Verification items for the finished model (mm, model axes). A direction names the side the tool comes from. Coordinates: 2 decimals unless noted, no trailing zeros. Write each loop counter-clockwise with the first axis right and the second up, starting at its lowest first coordinate (ties: lowest second). Pieces come first, ordered by that corner, then holes. Notation, with made-up numbers: (-23, 34.5) -> (17, 34.5) arc R14 cw to (17, 55.5) -> close; hole circle Ø1 at (-7, 28.5). An arc over 180 degrees is marked (long way). Answer in a Markdown table with one row per item.
```python
from build123d import *

# Parameters (mm, degrees)
F0_R     = 3.05
F0_R_2   = 1
F1_DEPTH = 12.5
F2_DEPTH = 12.5
F3_DEPTH = 14.8
F4_DEPTH = 14.1
F5_DEPTH = 22.2


with BuildPart() as f1:
    # F0 (on Front) → F1 (new body, symmetric)
    with BuildSketch(Plane.XZ):
        with BuildLine():
            Line((-3.724197, 20.562796), (-16.801276, 20.562796))
            ThreePointArc((-16.801276, 20.562796), (-20.212736, 13.062796), (-16.801276, 5.562796))
            Line((-16.801276, 5.562796), (-3.724197, 5.562796))
            ThreePointArc((-3.724197, 5.562796), (-0.312736, 13.062796), (-3.724197, 20.562796))
        make_face()
        with BuildLine():
            ThreePointArc((-13.092931, 9.062796), (-10.262736, 17.962796), (-7.432542, 9.062796))
            Line((-7.432542, 9.062796), (-13.092931, 9.062796))
        make_face(mode=Mode.SUBTRACT)
        with Locations((-10.262736, 13.062796)):
            Circle(F0_R)
        with Locations((-10.262736, 13.062796)):
            Circle(F0_R_2, mode=Mode.SUBTRACT)
        with BuildLine():
            Line((-13.092931, 9.062796), (-7.432542, 9.062796))
            ThreePointArc((-7.432542, 9.062796), (-10.262736, 17.962796), (-13.092931, 9.062796))
        make_face()
        with Locations((-10.262736, 13.062796)):
            Circle(F0_R, mode=Mode.SUBTRACT)
        with Locations((-10.262736, 13.062796)):
            Circle(F0_R_2)
    extrude(amount=F1_DEPTH, both=True)

    # F0 (on Front) → F2 (join)
    with BuildSketch(Plane.XZ):
        Polygon((-16.801197, 23.346301), (-16.801276, 20.562796), (-3.724197, 20.562796), (-3.724197, 23.346301), align=None)
    extrude(amount=F2_DEPTH)

    # F0 (on Front) → F3 (join)
    with BuildSketch(Plane.XZ):
        with BuildLine():
            Line((-13.092931, 9.062796), (-7.432542, 9.062796))
            ThreePointArc((-7.432542, 9.062796), (-10.262736, 17.962796), (-13.092931, 9.062796))
        make_face()
        with Locations((-10.262736, 13.062796)):
            Circle(F0_R, mode=Mode.SUBTRACT)
        with Locations((-10.262736, 13.062796)):
            Circle(F0_R)
        with Locations((-10.262736, 13.062796)):
            Circle(F0_R_2, mode=Mode.SUBTRACT)
        with Locations((-10.262736, 13.062796)):
            Circle(F0_R_2)
    extrude(amount=F3_DEPTH)

    # F0 (on Front) → F4 (join)
    with BuildSketch(Plane.XZ):
        with Locations((-10.262736, 13.062796)):
            Circle(F0_R)
        with Locations((-10.262736, 13.062796)):
            Circle(F0_R_2, mode=Mode.SUBTRACT)
    extrude(amount=-F4_DEPTH)

    # F0 (on Front) → F5 (join)
    with BuildSketch(Plane.XZ):
        with Locations((-10.262736, 13.062796)):
            Circle(F0_R_2)
    extrude(amount=-F5_DEPTH)


solid = f1.part
```
1. Sectioned sample at C-C, the plane z = 14.75. Record the cut outline in (x, y), and give its area (3 significant figures).
Findings below:
| item | result |
|---|---|
| outline | (-20.07, -12.5) -> (-14.86, -12.5) -> (-14.86, -14.8) -> (-5.66, -14.8) -> (-5.66, -12.5) -> (-0.46, -12.5) -> (-0.46, 12.5) -> (-7.72, 12.5) -> (-7.72, 14.1) -> (-12.8, 14.1) -> (-12.8, 12.5) -> (-20.07, 12.5) -> close |
| area | 520 mm² |
2. Sectioned sample at D-D, the plane z = 16.75. Record the cut outline in (x, y), and give its area (3 significant figures).
Findings below:
| item | result |
|---|---|
| outline | (-19.5, -12.5) -> (-13.49, -12.5) -> (-13.49, -14.8) -> (-7.04, -14.8) -> (-7.04, -12.5) -> (-1.02, -12.5) -> (-1.02, 12.5) -> (-19.5, 12.5) -> close |
| area | 477 mm² |
3. Sectioned sample at B-B, the plane x = -4.75. Record the cut outline in (y, z).
Findings below:
| item | result |
|---|---|
| outline | (-12.5, 5.56) -> (12.5, 5.56) -> (12.5, 20.56) -> (0, 20.56) -> (0, 23.35) -> (-12.5, 23.35) -> close |
4. Sectioned sample at A-A, the plane y = -1.5. Record the cut outline in (x, z), and give its area (3 significant figures).
Findings below:
| item | result |
|---|---|
| outline | (-16.8, 5.56) -> (-3.72, 5.56) arc R9.95 ccw to (-3.72, 20.56) -> (-3.72, 23.35) -> (-16.8, 23.35) -> (-16.8, 20.56) arc R9.95 ccw to start |
| area | 304 mm² |
5. Access from +Z, -Z, +X, -X, +Y, -Y to the whole of each face (thin tool, end or side, straight path). Record for faces 1 (the face through (-7.445, 13.289, 11.895)), 2 (the face through (-10, 6, 20.563)), 3 (the face through (-10.09, -13.63, 17.96)).
Findings below:
| item | result |
|---|---|
| face 1 | +Y |
| face 2 | +Z, +X, -X, +Y |
| face 3 | -Y |
6. Material ranges on probe 1 along Y at (x, z) = (-17.75, 11.25); probe 2 along X at (y, z) = (-0.5, 12.75); probe 3 along Y at (x, z) = (-8.5, 14.25), recorded low to high. Write a range as from..to.
Findings below:
| item | result |
|---|---|
| probe 1 | y = -12.5..12.5 |
| probe 2 | x = -20.21..-0.32 |
| probe 3 | y = -14.8..14.1 |
7. Go/stop test with flat-tipped pins: pin 1 (8 mm diameter, centred on x = -15, y = 6, fed in from +Z); pin 2 (1.4 mm diameter, centred on y = -4, z = 22.5, fed in from +X); pin 3 (10 mm diameter, centred on x = -7.5, z = 19, fed in from +Y); pin 4 (1.5 mm diameter, centred on y = 14.5, z = 18, fed in from +X). Record where each tip stops, or that it passes through.
Findings below:
| item | result |
|---|---|
| pin 1 | stops at z = 20.56 |
| pin 2 | stops at x = -3.72 |
| pin 3 | stops at y = 14.1 |
| pin 4 | passes through |
